For this review, take the finished solid that the model builds, in its own axes (mm). Round coordinates to 2 decimals unless told otherwise and drop trailing zeros. Loops run counter-clockwise (first coordinate to the right, second up) from the corner with the lowest first, then second, coordinate; pieces in that order, holes last. Notation, with made-up numbers: (5.25, 12) -> (34.25, 12) arc R18 ccw to (34.25, 38) -> close; hole circle Ø9 at (-6.75, 5.25). An arc over 180 degrees is marked (long way). Write each question's results on one line, items separated by ' | '.
```python
from build123d import *

# Parameters (mm, degrees)
F0_R     = 2.5
F1_DEPTH = 1.5


with BuildPart() as f1:
    # F0 (on Front) → F1 (new body)
    with BuildSketch(Plane.XZ):
        Polygon((-3, -2), (3, -2), (3, 2), (6.5, 2), (6.5, 37), (3, 37), (3, 39.2), (0, 39.2), (-3, 39.2), (-3, 37), (-6.5, 37), (-6.5, 2), (-3, 2), align=None)
        with Locations((-2.559623, 15.623519)):
            Circle(F0_R, mode=Mode.SUBTRACT)
        Polygon((2.101456, 8.201567), (0, 5.761865), (-2.101456, 8.201567), (0, 12.142628), align=None, mode=Mode.SUBTRACT)
        Polygon((-2.101456, 30.798433), (0, 33.238135), (2.101456, 30.798433), (0, 26.857372), align=None, mode=Mode.SUBTRACT)
    extrude(amount=F1_DEPTH)


solid = f1.part
```
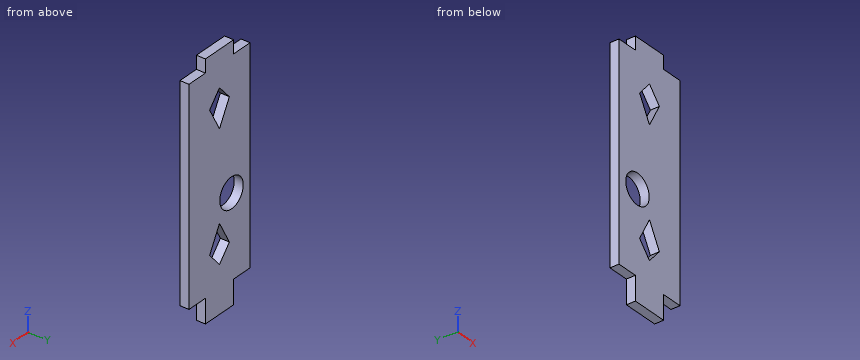
1. Consider section D-D (x = -3.5). State the section outline as (y, z) points, plus the area to 3 significant figures.
Values found:
outline: (-1.5, 2) -> (0, 2) -> (0, 13.31) -> (-1.5, 13.31) -> close; (-1.5, 17.94) -> (0, 17.94) -> (0, 37) -> (-1.5, 37) -> close | area: 45.6 mm2
2. To check wall thickness, follow probe 1 along Z at (x, y) = (-2, -0.3); probe 2 along Z at (x, y) = (-1.5, -0.1); probe 3 along Z at (x, y) = (5.75, -0.35). State the ranges of each line that lie inside material, in increasing order.
Values found:
probe 1: z = -2 to 8.08, 8.39 to 13.19, 18.06 to 30.61, 30.92 to 39.2 | probe 2: z = -2 to 7.5, 9.33 to 13.36, 17.89 to 29.67, 31.5 to 39.2 | probe 3: z = 2 to 37
3. Consider section B-B (y = -0.25). State the section outline as (x, z) points.
Values found:
outline: (-6.5, 2) -> (-3, 2) -> (-3, -2) -> (3, -2) -> (3, 2) -> (6.5, 2) -> (6.5, 37) -> (3, 37) -> (3, 39.2) -> (-3, 39.2) -> (-3, 37) -> (-6.5, 37) -> close; hole circle Ø5 at (-2.56, 15.62); hole (-2.1, 8.2) -> (0, 5.76) -> (2.1, 8.2) -> (0, 12.14) -> close; hole (-2.1, 30.8) -> (0, 26.86) -> (2.1, 30.8) -> (0, 33.24) -> close
4. Consider section C-C (x = -0.5). State the section outline as (y, z) points, plus the area to 3 significant figures.
Values found:
outline: (-1.5, -2) -> (0, -2) -> (0, 6.34) -> (-1.5, 6.34) -> close; (-1.5, 11.2) -> (0, 11.2) -> (0, 14.21) -> (-1.5, 14.21) -> close; (-1.5, 17.04) -> (0, 17.04) -> (0, 27.8) -> (-1.5, 27.8) -> close; (-1.5, 32.66) -> (0, 32.66) -> (0, 39.2) -> (-1.5, 39.2) -> close | area: 43.0 mm2
5. Consider section A-A (z = 6.5). State the section outline as (x, y) points, plus the area to 3 significant figures.
Values found:
outline: (-6.5, -1.5) -> (-0.64, -1.5) -> (-0.64, 0) -> (-6.5, 0) -> close; (0.64, -1.5) -> (6.5, -1.5) -> (6.5, 0) -> (0.64, 0) -> close | area: 17.6 mm2
6. For pin 1 (0.8 mm diameter, centred on x = 5.5, y = -1, fed in from -Z); pin 2 (0.8 mm diameter, centred on x = 4.5, y = -0.5, fed in from +Z); pin 3 (4.5 mm diameter, centred on x = -2.56, z = 15.62, fed in from -Y), all flat-tipped, find the tip position at first contact; note any pin that passes through.
Values found:
pin 1: stops at z = 2 | pin 2: stops at z = 37 | pin 3: passes through
